For this review, take the finished solid that the model builds, in its own axes (mm). Face numbers are marked on the shaded views. A direction names the side the tool comes from. Coordinates: 2 decimals unless noted, no trailing zeros. Order: outer loops, then holes, each group sorted by start corner. A loop starts at its lowest first (then second) coordinate and runs counter-clockwise, first axis right, second up. Notation, with made-up numbers: M 72,-22 L 91,-22 A24 cw 91,-8 Z; hole C 2.25,63 d7. An arc over 180 degrees is marked long. Use CSV: the item, a comma, the result in double quotes.
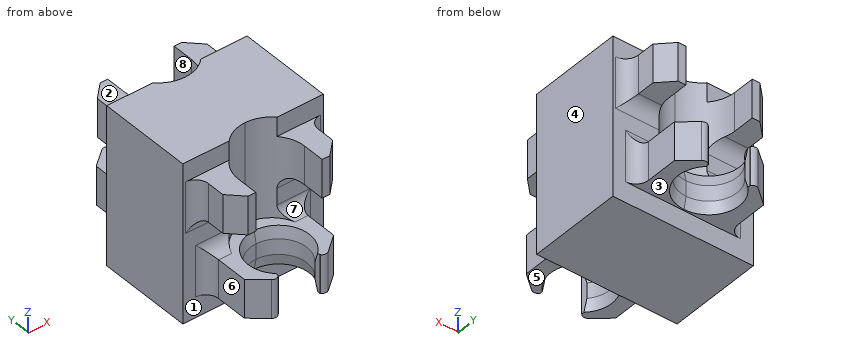
```python
from build123d import *

# Parameters (mm, degrees)
F1_DEPTH  = 12.4
F2_W      = 4.8141676475
F2_H      = 3.3
F2_H_2    = 1.6
F2_H_3    = 1.5
F3_DEPTH  = 25
F5_DEPTH  = 7.8
F6_DEPTH  = 0.8
F7_SIZE   = 1.1
F8_R      = 0.4
F9_R      = 1
F10_SIZE2 = 0.2
F10_SIZE  = 0.9


# Not quite as in the source:
# - a feature of the source that left no trace in its solid (it failed there, or was rolled back) is left out


with BuildPart() as f1:
    # F0 (on Top) → F1 (new body)
    with BuildSketch(Plane.XY):
        with BuildLine():
            ThreePointArc((0, -2.2), (-2.0110712703, -0.8919598342), (-1.6307225426, 1.476734231))
            Line((-1.6307225426, 1.476734231), (-1.6307225426, 1.976734231))
            Line((-1.6307225426, 1.976734231), (-1.9090909091, 2.3141676475))
            Line((-1.9090909091, 2.3141676475), (-3.5, 1.0017346067))
            Line((-3.5, 1.0017346067), (-3.5, -2.5))
            Line((-3.5, -2.5), (-5.5, -2.5))
            Line((-5.5, -2.5), (-5.5, -6.2))
            Line((-5.5, -6.2), (0, -6.2))
            Line((0, -6.2), (0, -2.2))
        make_face()
    extrude(amount=F1_DEPTH)

    # F2 (on face) → F3 (cut)
    with BuildSketch(Plane(origin=(-3.5, 0, 0), x_dir=(0, -1, 0), z_dir=(-1, 0, 0))):
        with Locations((0.0929161762, 6.25)):
            Rectangle(F2_W, F2_H)
        with Locations((0.0929161762, 0.8)):
            Rectangle(F2_W, F2_H_2)
        with Locations((0.0929161762, 11.65)):
            Rectangle(F2_W, F2_H_3)
    extrude(amount=-F3_DEPTH, mode=Mode.SUBTRACT)

    # F4 (on face) → F5 (cut, through all)
    with BuildSketch(Plane.XY.offset(12.4)):
        with BuildLine():
            Line((-2.6, 1.0017346067), (-2.6, -0.7))
            ThreePointArc((-2.6, -0.7), (-1.8384776311, -2.5384776311), (0, -3.3))
            Line((0, -3.3), (0, -2.2))
            ThreePointArc((0, -2.2), (-2.0110712703, -0.8919598342), (-1.6307225426, 1.476734231))
            Line((-1.6307225426, 1.476734231), (-1.6307225426, 1.976734231))
            Line((-1.6307225426, 1.976734231), (-1.9090909091, 2.3141676475))
            Line((-1.9090909091, 2.3141676475), (-3.5, 1.0017346067))
            Line((-3.5, 1.0017346067), (-2.6, 1.0017346067))
        make_face()
    extrude(amount=-F5_DEPTH, mode=Mode.SUBTRACT)

    # F6 (add): a face of the model
    f6_faces = [f1.faces().sort_by_distance(p)[0] for p in [
        (-3.5, -0.7491326967, 9.4),
    ]]
    extrude(f6_faces, amount=F6_DEPTH)

    # F7
    f7_edges = [f1.edges().sort_by_distance(p)[0] for p in [
        (-4.3, 1.001735, 9.4),
    ]]
    chamfer(f7_edges, length=F7_SIZE)

    # F8
    f8_edges = [f1.edges().sort_by_distance(p)[0] for p in [
        (-1.909091, 2.314168, 3.1),
    ]]
    fillet(f8_edges, radius=F8_R)

    # F9
    f9_edges = [f1.edges().sort_by_distance(p)[0] for p in [
        (-3.5, -2.5, 3.1),
        (-2.688083, -2.5, 4.6),
        (-3.088083, -2.5, 7.9),
        (-4.3, -2.5, 9.4),
    ]]
    fillet(f9_edges, radius=F9_R)

    # F10
    f10_edges = [f1.edges().sort_by_distance(p)[0] for p in [
        (-2.011071, -0.89196, 1.6),
        (-2.011071, -0.89196, 4.6),
    ]]
    f10_side = f1.faces().sort_by_distance((-2.011071, -0.89196, 3.1))[0]
    chamfer(f10_edges, length=F10_SIZE, length2=F10_SIZE2, reference=f10_side)

    # F11: F1 across face


with BuildPart() as f1_1:
    add(f1.part)
    add(f1.part.mirror(Plane(origin=(0, -4.5388751239, 5.7890981169), x_dir=(0, 1, 0), z_dir=(1, 0, 0))))

    # F12: F1 across face


with BuildPart() as f1_2:
    add(f1_1.part)
    add(f1_1.part.mirror(Plane(origin=(0, -6.2, 6.2), x_dir=(1, 0, 0), z_dir=(0, -1, 0))))


solid = f1_2.part
```
Item 1: Add section D-D on z = 10. State the section outline as (x, y) points.
Solutions:
outline,"M -5.5,-9.9 L -5.3,-9.9 A1 cw -4.3,-10.9 L -4.3,-12.3 L -3.2,-13.4 L -2.6,-13.4 L -2.6,-11.7 A2.6 cw 2.6,-11.7 L 2.6,-13.4 L 3.2,-13.4 L 4.3,-12.3 L 4.3,-10.9 A1 cw 5.3,-9.9 L 5.5,-9.9 L 5.5,-2.5 L 5.3,-2.5 A1 cw 4.3,-1.5 L 4.3,-0.1 L 3.2,1 L 2.6,1 L 2.6,-0.7 A2.6 cw -2.6,-0.7 L -2.6,1 L -3.2,1 L -4.3,-0.1 L -4.3,-1.5 A1 cw -5.3,-2.5 L -5.5,-2.5 Z"
Item 2: To check wall thickness, follow line 1 along X through (y, z) = (-12.25, 9.25); line 2 along Z through (x, y) = (3, -12); line 3 along Y through (x, z) = (-4.5, 11). State the ranges of each line that lie inside material, in increasing order. Write a range as [from, to].
Solutions:
line 1,"[-4.3, -2.6], [2.6, 4.3]"
line 2,"[1.6, 4.6], [7.9, 10.9]"
line 3,"[-9.9, -2.5]"
Item 3: Add section A-A on z = 6. State the section outline as (x, y) points.
Solutions:
outline,"M -5.5,-9.9 L -1.88,-9.9 A2.6 cw 1.88,-9.9 L 5.5,-9.9 L 5.5,-2.5 L 1.88,-2.5 A2.6 cw -1.88,-2.5 L -5.5,-2.5 Z"
Item 4: Add section C-C on y = -0.5. State how many separate pieces and enclosed holes the cut face has, and give its area (3 significant figures).
Solutions:
separate pieces,"4"
enclosed holes,"0"
area,"18.0 mm^2"
Item 5: Draft analysis for pull direction Z (two halves, no side actions). For the marked faces 1, 2, 3 and 4, state which applies: released by +Z, released by -Z, zero draft, split by the parting line, or undercut.
Solutions:
face 1,"undercut"
face 2,"released by +Z"
face 3,"released by -Z"
face 4,"zero draft"
Item 6: Clearance check with flat-ended pins moving along their axes: pin 1 Ø1 at (y, z) = (-12.5, 4.5) entering from -X; pin 2 Ø1 at (x, z) = (4, 10.5) entering from -Y; pin 3 Ø1.9 at (y, z) = (0.5, 9) entering from +X; pin 4 Ø1.6 at (x, y) = (0.5, -13) entering from +Z. State where each tip first meets the part, or that it passes through.
Solutions:
pin 1,"x = -3.5"
pin 2,"y = -13.1"
pin 3,"x = 4.3"
pin 4,"through"
Item 7: For the marked faces 5, 6, 7 and 8, list the 3-axis set-ups (+Z, -Z, +X, -X, +Y, -Y) from which the entire face can be reached by the end or side of a thin tool; tool diameter is ignored.
Solutions:
face 5,"-Z, +X, -X, -Y"
face 6,"-Z, -X, -Y"
face 7,"+X, -X, -Y"
face 8,"+Z, +Y"
